Geometry: final body of the model. Coordinates: model frame, mm. Face numbers are marked on the shaded views. Coordinates: 2 decimals unless noted, no trailing zeros. One line per item, written item: value. Start each with the question number.
Item 1: Mould query, pull axis Z, two halves, no side actions, for the marked faces 1 and 2. Classes: +Z half, -Z half, draft (parallel to the pull), parting line (faces both ways), or undercut.
Item 2: Section query A-A on z = -0.9. Give the number of separate pieces and of enclosed holes in the cut face, then the cut area to 3 significant figures.
Item 3: Ray query, probe 1 along X at (y, z) = (-38.5, -1.3); probe 2 along Y at (x, z) = (43, -0.4); probe 3 along Y at (x, z) = (59, -2.35). Return the intervals inside material, ascending. Write a range as from..to.
Item 4: Contact query for flat-ended pins moving along their axis: pin 1 Ø0.9 at (x, z) = (35.5, -1) entering from -Y; pin 2 Ø1.5 at (x, z) = (140.5, -2) entering from -Y; pin 3 Ø1.5 at (x, z) = (-51, -2) entering from +Y. Output: stop coordinate, or through.
from build123d import *

# Parameters (mm, degrees)
SKETCH1_RX          = 244
SKETCH1_RY          = 110
BOSS_EXTRUDE1_DEPTH = 3
CUT_EXTRUDE5_DEPTH  = 4
SKETCH13_W          = 71.2
SKETCH13_H          = 34.45
CUT_EXTRUDE7_DEPTH  = 4
SKETCH12_R          = 6.83635542
CUT_EXTRUDE8_DEPTH  = 4
CHAMFER1_SIZE       = 10


with BuildPart() as part:
    # Sketch1 → Boss-Extrude1 (new body)
    with BuildSketch(Plane.XY):
        with Locations((0, 0)):
            Ellipse(SKETCH1_RX, SKETCH1_RY)
    extrude(amount=-BOSS_EXTRUDE1_DEPTH)

    # Sketch10 → Cut-Extrude5 (cut, through all)
    with BuildSketch(Plane.XY):
        Polygon((-137.5, 83.1), (137.5, 83.1), (137.5, 28.1), (142.5, 28.1), (142.5, 25.1), (137.5, 25.1), (137.5, 15.1), (-137.5, 15.1), (-137.5, 25.1), (-142.5, 25.1), (-142.5, 28.1), (-137.5, 28.1), align=None)
    extrude(amount=-CUT_EXTRUDE5_DEPTH, mode=Mode.SUBTRACT)

    # Sketch13 → Cut-Extrude7 (cut, through all)
    with BuildSketch(Plane.XY):
        with Locations((-40.6, -32.225)):
            Rectangle(SKETCH13_W, SKETCH13_H)
        with Locations((-40.6, -76.675)):
            Rectangle(SKETCH13_W, SKETCH13_H)
        with Locations((40.6, -32.225)):
            Rectangle(SKETCH13_W, SKETCH13_H)
        with Locations((40.6, -76.675)):
            Rectangle(SKETCH13_W, SKETCH13_H)
    extrude(amount=-CUT_EXTRUDE7_DEPTH, mode=Mode.SUBTRACT)

    # Sketch12 → Cut-Extrude8 (cut, through all)
    with BuildSketch(Plane.XY):
        with Locations((200, -30)):
            Circle(SKETCH12_R)
        with Locations((-200, -30)):
            Circle(SKETCH12_R)
    extrude(amount=-CUT_EXTRUDE8_DEPTH, mode=Mode.SUBTRACT)

    # Chamfer1
    chamfer1_edges = [part.edges().sort_by_distance(p)[0] for p in [
        (-137.5, 83.1, -1.5),
        (137.5, 83.1, -1.5),
    ]]
    chamfer(chamfer1_edges, length=CHAMFER1_SIZE)


solid = part.part
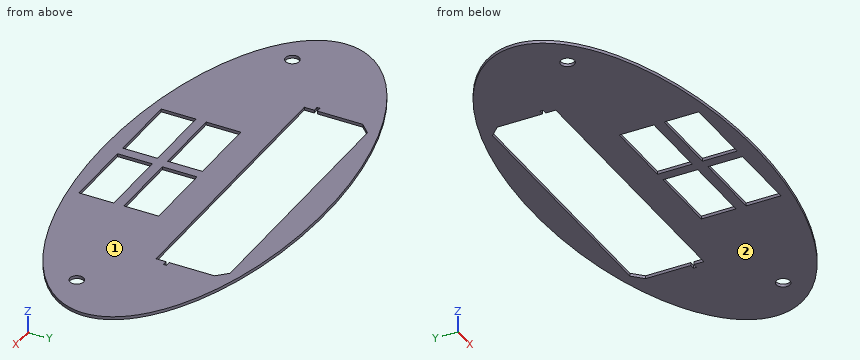
Reply:
1. face 1: +Z half
1. face 2: -Z half
2. separate pieces: 1
2. enclosed holes: 7
2. area: 55,600 mm²
3. probe 1: x = -228.57..-76.2, -5..5, 76.2..228.57
3. probe 2: y = -108.28..-93.9, -59.45..-49.45, -15..15.1, 83.1..108.28
3. probe 3: y = -106.74..-93.9, -59.45..-49.45, -15..15.1, 83.1..106.74
4. pin 1: stops at y = -108.86
4. pin 2: stops at y = -90.17
4. pin 3: stops at y = 107.64
